The listing builds one solid part. Answer for the finished solid, in the listing's coordinates (mm). A direction names the side the tool comes from. Give positions to 0.01 mm unless a question says otherwise; leave off trailing zeros. Loops run counter-clockwise (first coordinate to the right, second up) from the corner with the lowest first, then second, coordinate; pieces in that order, holes last. Notation, with made-up numbers: M -37.75,-17.75 L -26.75,-17.75 A23 cw -26.75,2.25 Z; hole C -29.75,20.25 d5. An arc over 180 degrees is marked long. One line per item, written item: value. Start each with the question number.
Q1. Flat-ended cylindrical pins translate along their axes: pin 1 (1.5 mm diameter, centred on x = 0.5, z = 0.5, fed in from +Y); pin 2 (1.5 mm diameter, centred on y = 3, z = -0.5, fed in from +X); pin 3 (1.1 mm diameter, centred on y = 4, z = -2, fed in from +X). Find the tip coordinate at first contact, or state that the pin passes through.
Q2. Consider L1, parallel to X at y = 2.8, z = -0.35; L2, parallel to X at y = 4, z = 0.6; L3, parallel to X at y = 0.65, z = 0.1. Determine where each line is inside the solid, lowest interval first.
Q3. A cutting plane is placed at D-D, the plane y = 4.7. Determine the outline of the cut face in (x, z), and give its area (3 significant figures).
Q4. A cutting plane is placed at C-C, the plane x = 1.2. Determine the outline of the cut face in (y, z).
Q5. For faces 4 (the flat face through (1.15, 1.91, 2.5)), 5 (the flat face through (-1, 4, -2)), 6 (the flat face through (0, 1, 0)), determine the directions among +Z, -Z, +X, -X, +Y, -Y from which every point of the face is accessible in a straight line to the end or side of a thin tool.
Q6. A cutting plane is placed at A-A, the plane y = 4.1. Determine the outline of the cut face in (x, z).
Q7. A cutting plane is placed at B-B, the plane z = -0.15. Determine the outline of the cut face in (x, y).
Q8. The mould has two halves that part along X. Classify faces 1 (the flat face through (2.5, 2, 0)), 2 (the flat face through (-1.5, 3, 0)), 3 (the flat face through (2, 5, 0)): +X half, -X half, draft (parallel to the pull), parting line (faces both ways), or undercut.
Autodesk Inventor part; units mm, degrees
ref_plane "YZ Plane" through (0, 0, 0) normal (1, 0, 0) x (0, 1, 0)
ref_plane "XZ Plane" through (0, 0, 0) normal (0, 1, 0) x (-1, 0, 0)
ref_plane "XY Plane" through (0, 0, 0) normal (0, 0, 1) x (1, 0, 0)
sketch "Sketch1" plane through (0, 0, 0) normal (0, 1, 0) x (-1, 0, 0)
  line L0 (-2.5, 2.5) -> (2.5, 2.5)
  line L1 (2.5, 2.5) -> (2.5, -2.5)
  line L2 (2.5, -2.5) -> (-2.5, -2.5)
  line L3 (-2.5, -2.5) -> (-2.5, 2.5)
  line L4 (-2.5, 2.5) -> (2.5, -2.5) construction
  line L5 (2.5, 2.5) -> (-2.5, -2.5) construction
  point P0 (0, 0)
  dimension "d0" = 5
  dimension "d1" = 5
extrude "Extrusion1" add sketch "Sketch1" along normal blind 5
shell "Shell1" thickness 1 removed faces 1 at (-0.8333, 5, -0.8333)
sketch "Sketch3" plane through (-2.5, 0, 2.5) normal (0, 0, 1) x (1, 0, 0)
  line L0 (2.5, 9.1674) -> (2.5, 2.1156) construction
  line L1 (1.4995, 9.1674) -> (1.4995, 2.1156)
  line L2 (3.5005, 2.1156) -> (3.5005, 9.1674)
  arc A0 (3.5005, 9.1674) -> (1.4995, 9.1674) centre (2.5, 9.1674) ccw
  arc A1 (1.4995, 2.1156) -> (3.5005, 2.1156) centre (2.5, 2.1156) ccw
  point P0 (2.5, 0)
  point P1 (2.5, 5.6415)
extrude "Extrusion3" cut sketch "Sketch3" against normal through all
sketch "Sketch4" plane through (0, 5, 0) normal (0, 1, 0) x (1, 0, 0)
  point P0 (0, 0)
sketch "Sketch5" plane through (0, 5, 0) normal (0, 1, 0) x (1, 0, 0)
  point P0 (0, 0)
sketch "Sketch6" plane through (0, 5, 0) normal (0, 1, 0) x (1, 0, 0)
  point P0 (0, 0)
sketch "Sketch7" plane through (0, 0, 0) normal (0, -1, 0) x (1, 0, 0)
  point P0 (0, 0)
sketch "Sketch8" plane through (-2.5, 0, -2.5) normal (-1, 0, 0) x (0, 0, 1)
  point P0 (2.5, 0)
sketch "Sketch9" plane through (2.5, 0, 2.5) normal (1, 0, 0) x (0, 0, -1)
  line L0 (1.5, 3.5) -> (3.5, 3.5)
  line L1 (3.5, 3.5) -> (3.5, 4.5)
  line L2 (3.5, 4.5) -> (1.5, 4.5)
  line L3 (1.5, 4.5) -> (1.5, 3.5)
  line L4 (1.5, 3.5) -> (3.5, 4.5) construction
  line L5 (3.5, 3.5) -> (1.5, 4.5) construction
  line L6 (0, 5) -> (5, 5)
  point P0 (2.5, 0)
  point P1 (2.5, 4)
  dimension "d10" = 1
  dimension "d14" = 2
  dimension "d15" = 1
extrude "Extrusion4" add sketch "Sketch9" along normal blind 0.5 draft -30
sketch "Sketch10" plane through (-2.5, 0, -2.5) normal (-1, 0, 0) x (0, 0, 1)
  line L0 (1.5, 3.5) -> (3.5, 3.5)
  line L1 (3.5, 3.5) -> (3.5, 4.5)
  line L2 (3.5, 4.5) -> (1.5, 4.5)
  line L3 (1.5, 4.5) -> (1.5, 3.5)
  line L4 (1.5, 3.5) -> (3.5, 4.5) construction
  line L5 (3.5, 3.5) -> (1.5, 4.5) construction
  line L6 (0, 5) -> (5, 5)
  point P0 (2.5, 0)
  point P1 (2.5, 4)
  dimension "d13" = 1
  dimension "d16" = 2
  dimension "d17" = 1
extrude "Extrusion5" add sketch "Sketch10" along normal blind 0.5 draft -30
equation "\"d16\" = d14"
equation "\"d17\" = d15"
properties part number "snapfit_v07"
Answer block:
1. pin 1: y = 1
1. pin 2: x = 2.93
1. pin 3: x = 2.5
2. L1: -2.5 to -1.5, 1.5 to 2.5
2. L2: -3 to -1.5, 1.5 to 3
2. L3: -2.5 to 2.5
3. outline: M -2.5,-2.5 L -1,-2.5 L -1,-1.5 L -1.5,-1.5 L -1.5,1.5 L -1,1.5 L -1,2.5 L -2.5,2.5 Z; M 1,-2.5 L 2.5,-2.5 L 2.5,2.5 L 1,2.5 L 1,1.5 L 1.5,1.5 L 1.5,-1.5 L 1,-1.5 Z
3. area: 12.0 mm^2
4. outline: M 0,-2.5 L 5,-2.5 L 5,-1.5 L 1,-1.5 L 1,1.5 L 5,1.5 L 5,2.5 L 0,2.5 Z
5. face 4: +Z, +X, -X, +Y, -Y
5. face 5: +Z, -Z, +Y
5. face 6: +Y
6. outline: M -3,-0.71 L -2.5,-1 L -2.5,-2.5 L -1,-2.5 L -1,-1.5 L -1.5,-1.5 L -1.5,1.5 L -1,1.5 L -1,2.5 L -2.5,2.5 L -2.5,1 L -3,0.71 Z; M 1,-2.5 L 2.5,-2.5 L 2.5,-1 L 3,-0.71 L 3,0.71 L 2.5,1 L 2.5,2.5 L 1,2.5 L 1,1.5 L 1.5,1.5 L 1.5,-1.5 L 1,-1.5 Z
7. outline: M -3,3.79 L -2.5,3.5 L -2.5,0 L 2.5,0 L 2.5,3.5 L 3,3.79 L 3,4.21 L 2.5,4.5 L 2.5,5 L 1.5,5 L 1.5,1 L -1.5,1 L -1.5,5 L -2.5,5 L -2.5,4.5 L -3,4.21 Z
8. face 1: +X half
8. face 2: undercut
8. face 3: draft
